from build123d import *

# Parameters (mm, degrees)
CROQUIS1_R              = 10
SALIENTE_EXTRUIR2_DEPTH = 80
CROQUIS4_R              = 25
SALIENTE_EXTRUIR3_DEPTH = 3
SALIENTE_EXTRUIR4_START = 25
CROQUIS5_R              = 25
SALIENTE_EXTRUIR4_DEPTH = 3
REDONDEO2_R             = 10
CORTAR_EXTRUIR1_START   = 80
CORTAR_EXTRUIR1_DEPTH   = 20
CORTAR_EXTRUIR2_START   = 80
CROQUIS7_W              = 3.5
CROQUIS7_H              = 7.2
CORTAR_EXTRUIR2_DEPTH   = 10
CORTAR_EXTRUIR3_START   = 1.785357468
CORTAR_EXTRUIR3_DEPTH   = 8.214642632
CORTAR_EXTRUIR4_START   = 24.165153
CROQUIS9_R              = 2
CORTAR_EXTRUIR4_DEPTH   = 3.834847


# Read off the part's stored shape, not the designer's step: Cortar-Extruir3
with BuildPart() as part:
    # Croquis1 → Saliente-Extruir2 (new body)
    with BuildSketch(Plane.XY):
        Circle(CROQUIS1_R)
    extrude(amount=SALIENTE_EXTRUIR2_DEPTH)

    # Croquis4 → Saliente-Extruir3 (add)
    with BuildSketch(Plane.XY):
        Circle(CROQUIS4_R)
    extrude(amount=SALIENTE_EXTRUIR3_DEPTH)

    # Croquis5 → Saliente-Extruir4 (add)
    with BuildSketch(Plane.XY.offset(SALIENTE_EXTRUIR4_START)):
        Circle(CROQUIS5_R)
    extrude(amount=SALIENTE_EXTRUIR4_DEPTH)

    # Redondeo2
    redondeo2_edges = [part.edges().sort_by_distance(p)[0] for p in [
        (-10, 0, 25),
        (-10, 0, 3),
    ]]
    fillet(redondeo2_edges, radius=REDONDEO2_R)

    # Croquis6 → Cortar-Extruir1 (cut)
    with BuildSketch(Plane.XY.offset(CORTAR_EXTRUIR1_START)):
        with BuildLine():
            Line((2, 1.5), (2, -1.5))
            ThreePointArc((2, -1.5), (-2.5, 0), (2, 1.5))
        make_face()
    extrude(amount=-CORTAR_EXTRUIR1_DEPTH, mode=Mode.SUBTRACT)

    # Croquis7 → Cortar-Extruir2 (cut)
    with BuildSketch(Plane.XY.offset(CORTAR_EXTRUIR2_START)):
        with Locations((5.5, 0)):
            Rectangle(CROQUIS7_W, CROQUIS7_H)
    extrude(amount=-CORTAR_EXTRUIR2_DEPTH, mode=Mode.SUBTRACT)

    # Cortar-Extruir3 outline → Cortar-Extruir3 (cut)
    with BuildSketch(Plane(origin=(0, 0, 0), x_dir=(0, 0, -1), z_dir=(1, 0, 0)).offset(CORTAR_EXTRUIR3_START)):
        with BuildLine():
            add(Edge.make_bspline(
                [(-73.250000008, 0), (-73.250010298, 0.457042806), (-73.439269311, 0.913556657), (-73.761440573, 1.236313288), (-74.083774062, 1.559232356), (-74.536167707, 1.749638189), (-74.998632957, 1.749999466), (-75.46109828, 1.75036072), (-75.914256207, 1.560125437), (-76.558728463, 0.916635921), (-76.75, 0.463408547), (-76.75, -0.463408547), (-76.559497121, -0.915462775), (-75.915045576, -1.559741953), (-75.458501248, -1.749734355), (-74.543528816, -1.750265056), (-74.088756627, -1.563446648), (-73.437067231, -0.912124478), (-73.250180582, -0.457964068), (-73.250000045, -0.000460382), (-73.250000003, -0.000230191), (-73.250000008, 0)],
                knots=[0.500062925, 0.500062925, 0.500062925, 0.500062925, 0.625, 0.625, 0.625000034, 0.750000005, 0.750000005, 0.750000019, 0.875000002, 0.875000002, 0.999999997, 0.999999997, 1.124999993, 1.124999993, 1.24999999, 1.24999999, 1.374999987, 1.374999987, 1.499999981, 1.499999981, 1.500062906, 1.500062906, 1.500062906, 1.500062906], degree=3))
        make_face()
    extrude(amount=CORTAR_EXTRUIR3_DEPTH, mode=Mode.SUBTRACT)

    # Croquis9 → Cortar-Extruir4 (cut)
    with BuildSketch(Plane.XY.offset(CORTAR_EXTRUIR4_START)):
        with Locations((18, 0)):
            Circle(CROQUIS9_R)
    extrude(amount=CORTAR_EXTRUIR4_DEPTH, mode=Mode.SUBTRACT)


solid = part.part
Work out the finished part from the listing and answer in its coordinate system (mm). A direction names the side the tool comes from. Round coordinates to 2 decimals unless told otherwise and drop trailing zeros. Loops run counter-clockwise (first coordinate to the right, second up) from the corner with the lowest first, then second, coordinate; pieces in that order, holes last. Notation, with made-up numbers: (-28, -21.5) -> (6, -21.5) arc R23 ccw to (6, 11.5) -> close; hole circle Ø5 at (43, 5.25). An arc over 180 degrees is marked (long way). Use one line per item in the form item = value.
(1) Flat-ended cylindrical pins translate along their axes: P1, Ø1.8, axis at x = 5, y = 1, coming from the +Z side; P2, Ø3.5, axis at y = -0.5, z = 70, coming from the -X side; P3, Ø3, axis at x = 4, z = 27, coming from the -Y side. Find the tip coordinate at first contact, or state that the pin passes through.
Answer list:
P1 = 70
P2 = -10
P3 = -24.87
(2) Find section C-C on z = 58. Give the vertices of the cut face in (x, y).
Answer list:
outline = circle Ø20 at (0, 0)
(3) Straight lines are drawn through the part: line 1 (X direction, y = 0, z = 71); line 2 (Z direction, x = 6, y = 21); line 3 (Y direction, x = 0, z = 65.5). For each, find the intervals that lie inside material, in ascending order.
Answer list:
line_1 = -10 to -2.5, 2 to 3.75, 7.25 to 10
line_2 = 0 to 3, 25 to 28
line_3 = -10 to -2.5, 2.5 to 10
(4) Find section A-A on x = 22.5. Give the vertices of the cut face in (y, z), then the cut area to 3 significant figures.
Answer list:
outline = (-10.9, 0) -> (10.9, 0) -> (10.9, 3) -> (-10.9, 3) -> close; (-10.9, 25) -> (10.9, 25) -> (10.9, 28) -> (-10.9, 28) -> close
area = 131 mm2
(5) A tool of negligible diameter and unlimited length cuts with its end or side. For faces 4 (the flat face through (5, 0, 70)), 5 (the flat face through (0, 0, 0)), 6 (the cylindrical face through (-2.17, -9.76, 13.99)), from which of +Z, -Z, +X, -X, +Y, -Y can it reach the whole face along a straight path? Write none if from no direction.
Answer list:
face_4 = +Z
face_5 = -Z, +X, -X, +Y, -Y
face_6 = none
(6) Find section B-B on x = 0. Give the vertices of the cut face in (y, z), then the cut area to 3 significant figures.
Answer list:
outline = (-25, 0) -> (25, 0) -> (25, 3) -> (20, 3) arc R10 cw to (10, 13) -> (10, 15) arc R10 cw to (20, 25) -> (25, 25) -> (25, 28) -> (10, 28) -> (10, 80) -> (2.5, 80) -> (2.5, 60) -> (-2.5, 60) -> (-2.5, 80) -> (-10, 80) -> (-10, 28) -> (-25, 28) -> (-25, 25) -> (-20, 25) arc R10 cw to (-10, 15) -> (-10, 13) arc R10 cw to (-20, 3) -> (-25, 3) -> close
area = 1,770 mm2
(7) Find section D-D on z = 11. Give the vertices of the cut face in (x, y), then the cut area to 3 significant figures.
Answer list:
outline = circle Ø20.4 at (0, 0)
area = 327 mm2
(8) For a pull along Y with two mould halves and no side action, classify faces 1 (the flat face through (-11, 17, 25)), 2 (the flat face through (5, 3.6, 75)), 3 (the cylindrical face through (23.846, 7.509, 1.479)) as released by +Y, released by -Y, zero draft, split by the parting line, or undercut.
Answer list:
face_1 = zero draft
face_2 = undercut
face_3 = split by the parting line
